from build123d import *

# Parameters (mm, degrees)
EXTRUDE_1_DEPTH     = 10
SKETCH_6_W          = 30
SKETCH_6_H          = 30
CUT_EXTRUDE_1_DEPTH = 4
SKETCH_7_W          = 30
SKETCH_7_H          = 30
CUT_EXTRUDE_2_DEPTH = 6
SKETCH_8_W          = 30
SKETCH_8_H          = 30
CUT_EXTRUDE_3_DEPTH = 8
CUT_EXTRUDE_4_DEPTH = 3


with BuildPart() as part:
    # 草图1 → 凸台-拉伸1 (new body)
    with BuildSketch(Plane.XY):
        with BuildLine():
            Line((62, -82.5), (-62, -82.5))
            ThreePointArc((-62, -82.5), (-64.121320344, -81.621320344), (-65, -79.5))
            Line((-65, -79.5), (-65, 79.5))
            ThreePointArc((-65, 79.5), (-64.121320344, 81.621320344), (-62, 82.5))
            Line((-62, 82.5), (62, 82.5))
            ThreePointArc((62, 82.5), (64.121320344, 81.621320344), (65, 79.5))
            Line((65, 79.5), (65, -79.5))
            ThreePointArc((65, -79.5), (64.121320344, -81.621320344), (62, -82.5))
        make_face()
    extrude(amount=EXTRUDE_1_DEPTH)

    # 草图6 → 切除-拉伸1 (cut)
    with BuildSketch(Plane.XY.offset(10)):
        with Locations((-40, 57.5)):
            Rectangle(SKETCH_6_W, SKETCH_6_H)
        with Locations((0, 57.5)):
            Rectangle(SKETCH_6_W, SKETCH_6_H)
        with Locations((40, 57.5)):
            Rectangle(SKETCH_6_W, SKETCH_6_H)
    extrude(amount=-CUT_EXTRUDE_1_DEPTH, mode=Mode.SUBTRACT)

    # 草图7 → 切除-拉伸2 (cut)
    with BuildSketch(Plane.XY.offset(10)):
        with Locations((-40, 17.5)):
            Rectangle(SKETCH_7_W, SKETCH_7_H)
        with Locations((0, 17.5)):
            Rectangle(SKETCH_7_W, SKETCH_7_H)
        with Locations((40, 17.5)):
            Rectangle(SKETCH_7_W, SKETCH_7_H)
    extrude(amount=-CUT_EXTRUDE_2_DEPTH, mode=Mode.SUBTRACT)

    # 草图8 → 切除-拉伸3 (cut)
    with BuildSketch(Plane.XY.offset(10)):
        with Locations((-40, -22.5)):
            Rectangle(SKETCH_8_W, SKETCH_8_H)
        with Locations((0, -22.5)):
            Rectangle(SKETCH_8_W, SKETCH_8_H)
        with Locations((40, -22.5)):
            Rectangle(SKETCH_8_W, SKETCH_8_H)
    extrude(amount=-CUT_EXTRUDE_3_DEPTH, mode=Mode.SUBTRACT)

    # 草图9 → 切除-拉伸4 (cut)
    with BuildSketch(Plane.XY.offset(10)):
        with BuildLine():
            Line((-55, -71.5), (-37, -71.5))
            Line((-37, -71.5), (-37, -56.5))
            ThreePointArc((-37, -56.5), (-46, -47.5), (-55, -56.5))
            Line((-55, -56.5), (-55, -71.5))
        make_face()
        with BuildLine():
            Line((-25, -56.5), (-25, -71.5))
            Line((-25, -71.5), (-7, -71.5))
            Line((-7, -71.5), (-7, -56.5))
            ThreePointArc((-7, -56.5), (-16, -47.5), (-25, -56.5))
        make_face()
        with BuildLine():
            Line((5, -56.5), (5, -71.5))
            Line((5, -71.5), (23, -71.5))
            Line((23, -71.5), (23, -56.5))
            ThreePointArc((23, -56.5), (14, -47.5), (5, -56.5))
        make_face()
        with BuildLine():
            Line((35, -56.5), (35, -71.5))
            Line((35, -71.5), (53, -71.5))
            Line((53, -71.5), (53, -56.5))
            ThreePointArc((53, -56.5), (44, -47.5), (35, -56.5))
        make_face()
    extrude(amount=-CUT_EXTRUDE_4_DEPTH, mode=Mode.SUBTRACT)


solid = part.part
Here's how the part is built. I have some questions about the finished solid (model axes, mm). Give positions to 0.01 mm unless a question says otherwise; leave off trailing zeros. Order: outer loops, then holes, each group sorted by start corner. A loop starts at its lowest first (then second) coordinate and runs counter-clockwise, first axis right, second up. Notation, with made-up numbers: (54.5, -36.75) -> (79.5, -36.75) arc R19 cw to (79.5, -10.75) -> close; hole circle Ø9 at (84.25, 73). An arc over 180 degrees is marked (long way). One line per item, written item: value. Start each with the question number.
1. Will these pins go through, and if not, where does the flat tip stop? pin 1 Ø1.5 at (x, y) = (-26.5, -28.5) entering from +Z; pin 2 Ø1.5 at (x, y) = (-41.5, 26.5) entering from +Z; pin 3 Ø6 at (x, y) = (15, -52.5) entering from +Z.
2. Imagine slicing it at C-C, the plane y = 67. List the corners of the cut face in (x, z) for me, plus the area to 3 significant figures.
3. Imagine slicing it at D-D, the plane x = -23. List the corners of the cut face in (y, z) for me.
4. I need wall thicknesses on probe 1 along X at (y, z) = (68.5, 9.5); probe 2 along Y at (x, z) = (8.5, 4.75); probe 3 along X at (y, z) = (-56.5, 8.5). Which ranges of each line are inside material? Lowest first, please. Write a range as from..to.
5. Imagine slicing it at A-A, the plane x = -46. List the corners of the cut face in (y, z) for me, plus the area to 3 significant figures.
6. Imagine slicing it at B-B, the plane y = -64. List the corners of the cut face in (x, z) for me.
7. We'd pull the mould along X, two halves only. Please class faces 1 (the face through (1, -82.5, 5)), 2 (the face through (-40, -7.5, 6)): released by +X, released by -X, zero draft, split by the parting line, or undercut.
Values follow:
1. pin 1: stops at z = 2
1. pin 2: stops at z = 4
1. pin 3: stops at z = 7
2. outline: (-65, 0) -> (65, 0) -> (65, 10) -> (55, 10) -> (55, 6) -> (25, 6) -> (25, 10) -> (15, 10) -> (15, 6) -> (-15, 6) -> (-15, 10) -> (-25, 10) -> (-25, 6) -> (-55, 6) -> (-55, 10) -> (-65, 10) -> close
2. area: 940 mm2
3. outline: (-82.5, 0) -> (82.5, 0) -> (82.5, 10) -> (-50.84, 10) -> (-50.84, 7) -> (-71.5, 7) -> (-71.5, 10) -> (-82.5, 10) -> close
4. probe 1: x = -65..-55, -25..-15, 15..25, 55..65
4. probe 2: y = -82.5..-37.5, -7.5..2.5, 32.5..82.5
4. probe 3: x = -65..-55, -37..-25, -7..5, 23..35, 53..65
5. outline: (-82.5, 0) -> (82.5, 0) -> (82.5, 10) -> (72.5, 10) -> (72.5, 6) -> (42.5, 6) -> (42.5, 10) -> (32.5, 10) -> (32.5, 4) -> (2.5, 4) -> (2.5, 10) -> (-7.5, 10) -> (-7.5, 2) -> (-37.5, 2) -> (-37.5, 10) -> (-47.5, 10) -> (-47.5, 7) -> (-71.5, 7) -> (-71.5, 10) -> (-82.5, 10) -> close
5. area: 1,040 mm2
6. outline: (-65, 0) -> (65, 0) -> (65, 10) -> (53, 10) -> (53, 7) -> (35, 7) -> (35, 10) -> (23, 10) -> (23, 7) -> (5, 7) -> (5, 10) -> (-7, 10) -> (-7, 7) -> (-25, 7) -> (-25, 10) -> (-37, 10) -> (-37, 7) -> (-55, 7) -> (-55, 10) -> (-65, 10) -> close
7. face 1: zero draft
7. face 2: undercut
